```python
from build123d import *

# Parameters (mm, degrees)
EXTRUDE_1_DEPTH     = 251
SKETCH_2_R          = 2.25
CUT_EXTRUDE_1_DEPTH = 2.5


with BuildPart() as part:
    # Эскиз1 → Бобышка-Вытянуть1 (new body)
    with BuildSketch(Plane.XY):
        Polygon((0, 0), (0, 18.5), (1.5, 18.5), (1.5, 0), (15.75, 0), (15.75, -1.5), (-14.25, -1.5), (-14.25, 0), align=None)
    extrude(amount=EXTRUDE_1_DEPTH)

    # Эскиз2 → Вырез-Вытянуть1 (cut, through all)
    with BuildSketch(Plane(origin=(0, 0, 0), x_dir=(1, 0, 0), z_dir=(0, 1, 0))):
        with Locations((-7.125, -10)):
            Circle(SKETCH_2_R)
        with Locations((8.625, -10)):
            Circle(SKETCH_2_R)
        with Locations((-7.125, -241)):
            Circle(SKETCH_2_R)
        with Locations((8.625, -241)):
            Circle(SKETCH_2_R)
    extrude(amount=-CUT_EXTRUDE_1_DEPTH, mode=Mode.SUBTRACT)


solid = part.part
```
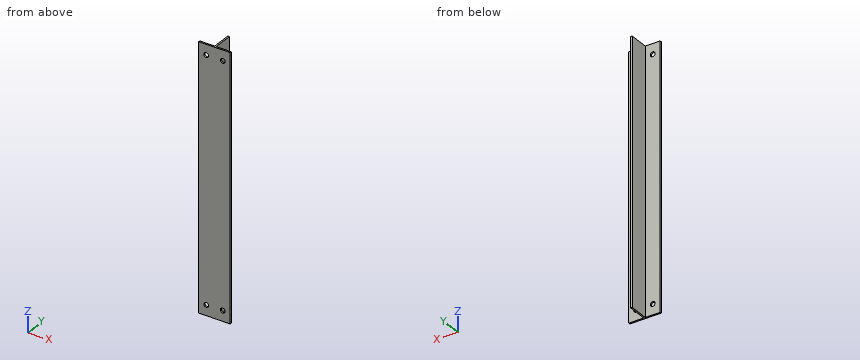
Source: CAD feature listing. Evaluate the final solid. Frame: model axes, mm. Coordinates: 2 decimals unless noted, no trailing zeros. Loops run counter-clockwise (first coordinate to the right, second up) from the corner with the lowest first, then second, coordinate; pieces in that order, holes last. Notation, with made-up numbers: M 76.25,77.25 L 110.25,77.25 A9 cw 110.25,91.25 Z; hole C 22,87 d4. An arc over 180 degrees is marked long. Use a Markdown table: item, result. Add a question column.
Q1. Section query A-A, the plane z = 241. Return loops of the section in (x, y) (3 decimals), and give its area (4 significant figures).
Q2. Section query B-B, the plane z = 185.5. Return loops of the section in (x, y).
Q3. Material intervals for L1, parallel to X at y = -0.85, z = 10 (3 decimals); L2, parallel to X at y = 16.25, z = 60; L3, parallel to Y at x = 4.75, z = 29, sorted ascending.
Q4. First-contact query: pin 1 (15.5 mm diameter, centred on x = -9.5, z = 114, fed in from +Y); pin 2 (4 mm diameter, centred on y = 15.5, z = 98.5, fed in from +X); pin 3 (3 mm diameter, centred on y = 15, z = 65, fed in from -X). Flat tips, straight axial feed; report the tip coordinate or a pass-through.
Q5. Section query C-C, the plane y = 13.5. Return loops of the section in (x, z), and give its area (4 significant figures).
Result:
| question | item | result |
|---|---|---|
| 1 | outline | M -14.25,-1.5 L -9.375,-1.5 L -9.375,0 L -14.25,0 Z; M -4.875,-1.5 L 6.375,-1.5 L 6.375,0 L 1.5,0 L 1.5,18.5 L 0,18.5 L 0,0 L -4.875,0 Z; M 10.875,-1.5 L 15.75,-1.5 L 15.75,0 L 10.875,0 Z |
| 1 | area | 59.25 mm2 |
| 2 | outline | M -14.25,-1.5 L 15.75,-1.5 L 15.75,0 L 1.5,0 L 1.5,18.5 L 0,18.5 L 0,0 L -14.25,0 Z |
| 3 | L1 | x = -14.25 to -9.375, -4.875 to 6.375, 10.875 to 15.75 |
| 3 | L2 | x = 0 to 1.5 |
| 3 | L3 | y = -1.5 to 0 |
| 4 | pin 1 | stops at y = 0 |
| 4 | pin 2 | stops at x = 1.5 |
| 4 | pin 3 | stops at x = 0 |
| 5 | outline | M 0,0 L 1.5,0 L 1.5,251 L 0,251 Z |
| 5 | area | 376.5 mm2 |
